For this review, take the finished solid that the model builds, in its own axes (mm). Face numbers are marked on the shaded views. A direction names the side the tool comes from. Coordinates: 2 decimals unless noted, no trailing zeros. Loops run counter-clockwise (first coordinate to the right, second up) from the corner with the lowest first, then second, coordinate; pieces in that order, holes last. Notation, with made-up numbers: M 44.5,-27 L 81.5,-27 A27 cw 81.5,9 Z; hole C -38,-16 d8. An arc over 180 degrees is marked long. Put each result on its own line as item: value.
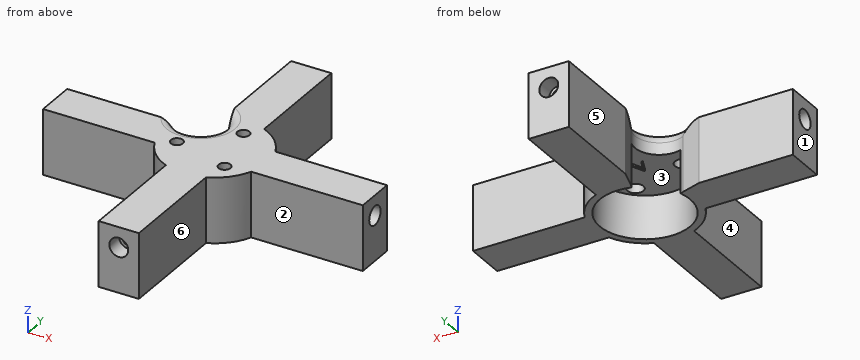
```python
from build123d import *

# Parameters (mm, degrees)
BOSS_EXTRUDE1_DEPTH     = 22.7
SKETCH5_R               = 1.5
CUT_EXTRUDE1_DEPTH      = 70
SKETCH6_R               = 11.25
CUT_EXTRUDE3_DEPTH      = 17.25
CUT_EXTRUDE3_DEPTH_BACK = 17.25
SKETCH7_R               = 2
CUT_EXTRUDE4_DEPTH      = 3
SKETCH8_W               = 6.5
SKETCH8_H               = 79.6
CUT_EXTRUDE5_DEPTH      = 58
CUT_EXTRUDE5_DEPTH_BACK = 66
SKETCH9_R               = 2.35
SKETCH9_R_2             = 1.55
CUT_EXTRUDE7_DEPTH      = 4
SKETCH9_3_R             = 1.55
CUT_EXTRUDE20_DEPTH     = 12
SKETCH21_R              = 2.35
SKETCH21_R_2            = 1.55
CUT_EXTRUDE22_DEPTH     = 4
SKETCH21_2_R            = 1.55
CUT_EXTRUDE23_DEPTH     = 12
SKETCH19_R              = 2.35
SKETCH19_R_2            = 1.55
CUT_EXTRUDE24_DEPTH     = 4
SKETCH19_2_R            = 1.55
CUT_EXTRUDE25_DEPTH     = 12
SKETCH20_R              = 2.35
SKETCH20_R_2            = 1.55
CUT_EXTRUDE26_DEPTH     = 4
SKETCH20_2_R            = 1.55
CUT_EXTRUDE27_DEPTH     = 12
FILLET2_R               = 2.5
BOSS_EXTRUDE2_DEPTH     = 0.5


with BuildPart() as part:
    # Sketch4 → Boss-Extrude1 (new body)
    with BuildSketch(Plane.XY):
        with BuildLine():
            Line((-5, 39.8), (-5, 12))
            ThreePointArc((-5, 12), (-9.192388155, 9.192388155), (-12, 5))
            Line((-12, 5), (-39.8, 5))
            Line((-39.8, 5), (-39.8, -5))
            Line((-39.8, -5), (-12, -5))
            ThreePointArc((-12, -5), (-9.192388155, -9.192388155), (-5, -12))
            Line((-5, -12), (-5, -39.8))
            Line((-5, -39.8), (5, -39.8))
            Line((5, -39.8), (5, -12))
            ThreePointArc((5, -12), (9.192388155, -9.192388155), (12, -5))
            Line((12, -5), (39.8, -5))
            Line((39.8, -5), (39.8, 5))
            Line((39.8, 5), (12, 5))
            ThreePointArc((12, 5), (9.192388155, 9.192388155), (5, 12))
            Line((5, 12), (5, 39.8))
            Line((5, 39.8), (-5, 39.8))
        make_face()
    extrude(amount=-BOSS_EXTRUDE1_DEPTH)

    # Sketch5 → Cut-Extrude1 (cut)
    with BuildSketch(Plane.XY):
        with Locations((2.184887392, 8.154110756)):
            Circle(SKETCH5_R)
        with Locations((-8.154110756, -2.184887392)):
            Circle(SKETCH5_R)
        with Locations((5.969223364, -5.969223364)):
            Circle(SKETCH5_R)
        with BuildLine():
            Line((-5, 16.456455054), (-3.523070126, 11.621395871))
            ThreePointArc((-3.523070126, 11.621395871), (-4.596194078, 4.596194078), (-11.621395871, 3.523070126))
            Line((-11.621395871, 3.523070126), (-16.456455054, 5))
            Line((-16.456455054, 5), (-14.526937175, 6.929517879))
            ThreePointArc((-14.526937175, 6.929517879), (-13.081475452, 13.081475452), (-6.929517879, 14.526937175))
            Line((-6.929517879, 14.526937175), (-5, 16.456455054))
        make_face()
    extrude(amount=-CUT_EXTRUDE1_DEPTH, mode=Mode.SUBTRACT)

    # Sketch6 → Cut-Extrude3 (cut, two sides)
    with BuildSketch(Plane(origin=(0, 0, -22.7), x_dir=(-1, 0, 0), z_dir=(0, 0, -1))) as cut_extrude3_sk:
        Circle(SKETCH6_R)
    extrude(amount=CUT_EXTRUDE3_DEPTH, mode=Mode.SUBTRACT)
    extrude(cut_extrude3_sk.sketch, amount=-CUT_EXTRUDE3_DEPTH_BACK, mode=Mode.SUBTRACT)

    # Sketch7 → Cut-Extrude4 (cut)
    with BuildSketch(Plane(origin=(0, 0, -5.45), x_dir=(-1, 0, 0), z_dir=(0, 0, -1))):
        with Locations((-2.184887392, 8.154110756)):
            Circle(SKETCH7_R)
        with Locations((-5.969223364, -5.969223364)):
            Circle(SKETCH7_R)
        with Locations((8.154110756, -2.184887392)):
            Circle(SKETCH7_R)
    extrude(amount=-CUT_EXTRUDE4_DEPTH, mode=Mode.SUBTRACT)

    # Sketch8 → Cut-Extrude5 (cut, two sides)
    with BuildSketch(Plane.ZY.offset(5)) as cut_extrude5_sk:
        with Locations((-19.45, 0)):
            Rectangle(SKETCH8_W, SKETCH8_H)
    extrude(amount=CUT_EXTRUDE5_DEPTH, mode=Mode.SUBTRACT)
    extrude(cut_extrude5_sk.sketch, amount=-CUT_EXTRUDE5_DEPTH_BACK, mode=Mode.SUBTRACT)

    # Sketch9 → Cut-Extrude7 (cut)
    with BuildSketch(Plane(origin=(0, 39.8, 0), x_dir=(1, 0, 0), z_dir=(0, 1, 0))):
        with Locations((0, 5)):
            Circle(SKETCH9_R)
        with Locations((0, 5)):
            Circle(SKETCH9_R_2, mode=Mode.SUBTRACT)
    extrude(amount=-CUT_EXTRUDE7_DEPTH, mode=Mode.SUBTRACT)

    # Sketch9_3 → Cut-Extrude20 (cut)
    with BuildSketch(Plane(origin=(0, 39.8, 0), x_dir=(1, 0, 0), z_dir=(0, 1, 0))):
        with Locations((0, 5)):
            Circle(SKETCH9_3_R)
    extrude(amount=-CUT_EXTRUDE20_DEPTH, mode=Mode.SUBTRACT)

    # Sketch21 → Cut-Extrude22 (cut)
    with BuildSketch(Plane.ZY.offset(39.8)):
        with Locations((-5, 0)):
            Circle(SKETCH21_R)
        with Locations((-5, 0)):
            Circle(SKETCH21_R_2, mode=Mode.SUBTRACT)
    extrude(amount=-CUT_EXTRUDE22_DEPTH, mode=Mode.SUBTRACT)

    # Sketch21_2 → Cut-Extrude23 (cut)
    with BuildSketch(Plane.ZY.offset(39.8)):
        with Locations((-5, 0)):
            Circle(SKETCH21_2_R)
    extrude(amount=-CUT_EXTRUDE23_DEPTH, mode=Mode.SUBTRACT)

    # Sketch19 → Cut-Extrude24 (cut)
    with BuildSketch(Plane(origin=(39.8, 0, 0), x_dir=(0, 0, -1), z_dir=(1, 0, 0))):
        with Locations((5, 0)):
            Circle(SKETCH19_R)
        with Locations((5, 0)):
            Circle(SKETCH19_R_2, mode=Mode.SUBTRACT)
    extrude(amount=-CUT_EXTRUDE24_DEPTH, mode=Mode.SUBTRACT)

    # Sketch19_2 → Cut-Extrude25 (cut)
    with BuildSketch(Plane(origin=(39.8, 0, 0), x_dir=(0, 0, -1), z_dir=(1, 0, 0))):
        with Locations((5, 0)):
            Circle(SKETCH19_2_R)
    extrude(amount=-CUT_EXTRUDE25_DEPTH, mode=Mode.SUBTRACT)

    # Sketch20 → Cut-Extrude26 (cut)
    with BuildSketch(Plane.XZ.offset(39.8)):
        with Locations((0, -5)):
            Circle(SKETCH20_R)
        with Locations((0, -5)):
            Circle(SKETCH20_R_2, mode=Mode.SUBTRACT)
    extrude(amount=-CUT_EXTRUDE26_DEPTH, mode=Mode.SUBTRACT)

    # Sketch20_2 → Cut-Extrude27 (cut)
    with BuildSketch(Plane.XZ.offset(39.8)):
        with Locations((0, -5)):
            Circle(SKETCH20_2_R)
    extrude(amount=-CUT_EXTRUDE27_DEPTH, mode=Mode.SUBTRACT)

    # Fillet2
    fillet2_edges = [part.edges().sort_by_distance(p)[0] for p in [
        (-4.596194078, 4.596194078, 0),
    ]]
    fillet(fillet2_edges, radius=FILLET2_R)

    # Sketch22 → Boss-Extrude2 (add)
    with BuildSketch(Plane(origin=(0, 0, -5.45), x_dir=(-1, 0, 0), z_dir=(0, 0, -1))):
        Polygon((-1.363621795, 3.175), (-1.058333333, 3.175), (0, 0.672906651), (1.058333333, 3.175), (1.363621795, 3.175), (0.020352564, 0), (-0.020352564, 0), align=None)
    extrude(amount=BOSS_EXTRUDE2_DEPTH)


solid = part.part
```
(1) Add section C-C (z = -12). Write out the cut boundary in (x, y), plus the area to 3 significant figures.
Determined:
outline: M -39.8,-5 L -12,-5 A13 ccw -5,-12 L -5,-39.8 L 5,-39.8 L 5,-12 A13 ccw 12,-5 L 39.8,-5 L 39.8,5 L 12,5 A13 ccw 5,12 L 5,39.8 L -5,39.8 L -5,16.46 L -3.52,11.62 A6 cw -3.17,10.8 A11.25 cw long -10.8,3.17 A6 cw -11.62,3.52 L -16.46,5 L -39.8,5 Z
area: 1,190 mm^2
(2) Draft analysis for pull direction Y (two halves, no side actions). For the marked faces 1, 2 and 3, state which applies: +Y half, -Y half, draft (parallel to the pull), parting line (faces both ways), or undercut.
Determined:
face 1: draft
face 2: -Y half
face 3: undercut
(3) Add section D-D (x = 14). Write out the cut boundary in (y, z).
Determined:
outline: M -5,-16.2 L 5,-16.2 L 5,0 L -5,0 Z
(4) Tool access review of the marked faces 4, 5 and 6: name each direction out of +Z, -Z, +X, -X, +Y, -Y from which nothing blocks a thin tool from reaching the whole face with its end or side.
Determined:
face 4: +Z, -Z, -X, -Y
face 5: +Z, -Z, -X, +Y
face 6: +Z, -Z, +X, -Y
(5) Add section B-B (x = 29). Write out the cut boundary in (y, z), plus the area to 3 significant figures.
Determined:
outline: M -5,-16.2 L 5,-16.2 L 5,0 L -5,0 Z; hole C 0,-5 d3.1
area: 154 mm^2
(6) For pin 1 (3 mm diameter, centred on x = 2.5, y = 9, fed in from -Z); pin 2 (6 mm diameter, centred on y = -24, z = -14, fed in from -X); pin 3 (4 mm diameter, centred on x = 0, z = -5, fed in from +Y), all flat-tipped, find the tip position at first contact; note any pin that passes through.
Determined:
pin 1: stops at z = -5.45
pin 2: stops at x = -5
pin 3: stops at y = 35.8
(7) Wall thickness on line 1 along X through (y, z) = (38.05, -5); line 2 along Z through (x, y) = (0, 29): over which ranges is each line inside the solid? List them lowest first. Write a range as [from, to].
Determined:
line 1: x = [-5, -2.35], [2.35, 5]
line 2: z = [-16.2, -6.55], [-3.45, 0]
(8) Add section A-A (z = -1). Write out the cut boundary in (x, y).
Determined:
outline: M -39.8,-5 L -12,-5 A13 ccw -5,-12 L -5,-39.8 L 5,-39.8 L 5,-12 A13 ccw 12,-5 L 39.8,-5 L 39.8,5 L 12,5 A13 ccw 5,12 L 5,39.8 L -5,39.8 L -5,16.46 L -4,13.18 A6.5 cw -13.18,4 L -16.46,5 L -39.8,5 Z; hole C -8.15,-2.18 d3; hole C 2.18,8.15 d3; hole C 5.97,-5.97 d3
